Solid Edge part; units mm, degrees
sketch "Sketch1" plane through (0, 0, 0) normal (0, 0, 1) x (1, 0, 0)
  arc A0 (-62.7617, -16.9107) -> (-57.8743, 29.59) centre (0, 0) cw
  line L0 (-45.07, 16.7858) -> (-57.8743, 29.59)
  line L1 (-45.07, 16.7858) -> (-16.7858, 45.07)
  line L2 (-16.7858, 45.07) -> (-29.59, 57.8743)
  arc A1 (-29.59, 57.8743) -> (29.59, 57.8743) centre (0, 0) cw
  line L3 (16.7858, 45.07) -> (29.59, 57.8743)
  line L4 (16.7858, 45.07) -> (45.07, 16.7858)
  line L5 (45.07, 16.7858) -> (57.8743, 29.59)
  arc A2 (57.8743, 29.59) -> (62.7617, -16.9107) centre (0, 0) cw
  line L6 (47.5751, -7.0484) -> (62.7617, -16.9107)
  line L7 (47.5751, -7.0484) -> (25.7895, -40.5952)
  line L8 (25.7895, -40.5952) -> (35.3554, -46.8074)
  line L9 (-35.3554, -46.8074) -> (35.3554, -46.8074)
  line L10 (-25.7895, -40.5952) -> (-35.3554, -46.8074)
  line L11 (-25.7895, -40.5952) -> (-47.5751, -7.0484)
  line L12 (-47.5751, -7.0484) -> (-62.7617, -16.9107)
extrude "ProtrusiónExtruida_1" add sketch "Sketch1" along normal mid plane 5
fillet "Round1" [suppressed]
hole "Agujero_1" at (-13.2502, 27.3924, 2.5) direction (0, 0, -1) diameter 3.2 end up to next
hole "Hole1" at (-27.3924, 13.2502, 2.5) direction (0, 0, -1) diameter 3.2 end up to next
hole "Hole2" at (-29.5486, -7.2655, 2.5) direction (0, 0, -1) diameter 3.2 end up to next
hole "Hole3" at (-18.6559, -24.0389, 2.5) direction (0, 0, -1) diameter 3.2 end up to next
hole "Hole4" at (13.2502, 27.3924, 2.5) direction (0, 0, -1) diameter 3.2 end up to next
hole "Hole5" at (27.3924, 13.2502, 2.5) direction (0, 0, -1) diameter 3.2 end up to next
hole "Hole6" at (29.5486, -7.2655, 2.5) direction (0, 0, -1) diameter 3.2 end up to next
hole "Hole7" at (18.6559, -24.0389, 2.5) direction (0, 0, -1) diameter 3.2 end up to next
fillet "Redondeo_4" radius 3 6 edges at (-62.7617, -16.9107, 0) (29.59, 57.8743, 0) (62.7617, -16.9107, 0) (57.8743, 29.59, 0) (-57.8743, 29.59, 0) (-29.59, 57.8743, 0)
hole "Agujero_9" at (0, 0, 2.5) direction (0, 0, -1) diameter 10 end up to next
Build history of the part. All positions in model axes, mm. A direction names the side the tool comes from. Give positions to 0.01 mm unless a question says otherwise; leave off trailing zeros. Order: outer loops, then holes, each group sorted by start corner. A loop starts at its lowest first (then second) coordinate and runs counter-clockwise, first axis right, second up. Notation, with made-up numbers: M -1,-36.75 L 56,-36.75 A12 ccw 56,-13.75 Z; hole C 4.25,60.25 d2. An arc over 180 degrees is marked long. Use one line per item in the form item = value.
1) Saw through at B-B (x = 0). Give the cut face in (y, z), plus the area to 3 significant figures.
Calculated:
outline = M -46.81,-2.5 L -5,-2.5 L -5,2.5 L -46.81,2.5 Z; M 5,-2.5 L 65,-2.5 L 65,2.5 L 5,2.5 Z
area = 509 mm2
2) Saw through at D-D (y = 50.5). Give the cut face in (x, z).
Calculated:
outline = M -22.22,-2.5 L 22.22,-2.5 L 22.22,2.5 L -22.22,2.5 Z
3) Two-plate mould, pull along Y, no slides. Class faces 6 (the face through (-21.61, 49.894, -0.035)), 7 (the face through (-49.894, 21.61, -0.035)), 8 (the face through (-64.672, 6.522, -0.035)): released by +Y, released by -Y, zero draft, split by the parting line, or undercut.
Calculated:
face_6 = undercut
face_7 = released by +Y
face_8 = split by the parting line
4) Tool access for faces 1 (the face through (30.73, 31.126, -0.035)), 2 (the face through (21.61, 49.894, -0.035)), 3 (the face through (-53.296, -10.764, -0.035)), 4 (the face through (49.894, 21.61, -0.035)), 5 (the face through (-30.51, -43.66, -0.04)): list every direction of +Z, -Z, +X, -X, +Y, -Y with a clear straight run to the whole face (end or side of a thin tool).
Calculated:
face_1 = +Z, -Z
face_2 = +Z, -Z, +X
face_3 = +Z, -Z, -Y
face_4 = +Z, -Z, +Y
face_5 = +Z, -Z, -X
5) Saw through at C-C (z = 0.6). State how many separate pieces and enclosed holes the cut face has, plus the area to 3 significant figures.
Calculated:
separate_pieces = 1
enclosed_holes = 9
area = 8,780 mm2
6) Probe probe 1 along X at (y, z) = (12, 1.45); probe 2 along Y at (x, z) = (-19, -2.15); probe 3 along Y at (x, z) = (32.5, 0.55). List the from-to ranges inside material, lowest first.
Calculated:
probe_1 = -63.88 to -28.39, -26.39 to 26.39, 28.39 to 63.88
probe_2 = -46.81 to -25.6, -22.48 to 42.86, 47.28 to 62.16
probe_3 = -46.81 to -44.95, -30.26 to 29.36
7) Drop flat-ended pins along their axis: pin 1 (3 mm diameter, centred on x = -17, z = 1, fed in from +Y); pin 2 (1.5 mm diameter, centred on x = -48, z = 1, fed in from -Y); pin 3 (3 mm diameter, centred on y = 51, z = -1, fed in from +X). Give the stop position or say it passes through.
Calculated:
pin_1 = 63.12
pin_2 = -7.81
pin_3 = 24.22
8) Saw through at A-A (y = 0). Give the cut face in (x, z).
Calculated:
outline = M -65,-2.5 L -5,-2.5 L -5,2.5 L -65,2.5 Z; M 5,-2.5 L 65,-2.5 L 65,2.5 L 5,2.5 Z
